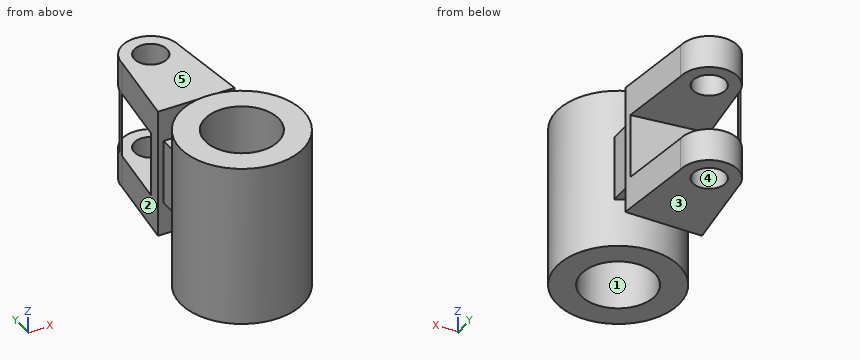
from build123d import *

# Parameters (mm, degrees)
SKETCH1_R           = 37.5
SKETCH1_R_2         = 22.5
BOSS_EXTRUDE1_DEPTH = 50
BOSS_EXTRUDE3_DEPTH = 40
SKETCH10_R          = 10
CUT_EXTRUDE5_DEPTH  = 91
SKETCH11_W          = 40
SKETCH11_H          = 59.943754609
CUT_EXTRUDE6_DEPTH  = 71.990693952
SKETCH12_W          = 40
SKETCH12_H          = 20
BOSS_EXTRUDE8_DEPTH = 20


with BuildPart() as part:
    # Sketch1 → Boss-Extrude1 (new body, symmetric)
    with BuildSketch(Plane.XY):
        Circle(SKETCH1_R)
        Circle(SKETCH1_R_2, mode=Mode.SUBTRACT)
    extrude(amount=BOSS_EXTRUDE1_DEPTH, both=True)



with BuildPart() as body_2:
    # Sketch3 → Boss-Extrude3 (new body, symmetric)
    with BuildSketch(Plane.XY):
        with BuildLine():
            Line((-23.5, 50), (23.5, 50))
            Line((23.5, 50), (17.5, 100))
            ThreePointArc((17.5, 100), (0, 117.5), (-17.5, 100))
            Line((-17.5, 100), (-23.5, 50))
        make_face()
    extrude(amount=BOSS_EXTRUDE3_DEPTH, both=True)

    # Sketch10 → Cut-Extrude5 (cut, through all)
    with BuildSketch(Plane.XY.offset(40)):
        with Locations((0, 100)):
            Circle(SKETCH10_R)
    extrude(amount=-CUT_EXTRUDE5_DEPTH, mode=Mode.SUBTRACT)

    # Sketch11 → Cut-Extrude6 (cut, through all)
    with BuildSketch(Plane(origin=(-29.081230284, 3.489747634, 0), x_dir=(0, 0, 1), z_dir=(-0.992876838, 0.119145221, 0))):
        with Locations((0, 86.815806545)):
            Rectangle(SKETCH11_W, SKETCH11_H)
    extrude(amount=-CUT_EXTRUDE6_DEPTH, mode=Mode.SUBTRACT)


with BuildPart() as part_1:
    add(part.part)

    add(body_2.part)  # Boss-Extrude8 merges body 2
    # Sketch12 → Boss-Extrude8 (add, symmetric)
    with BuildSketch(Plane.XY):
        with Locations((0, 40)):
            Rectangle(SKETCH12_W, SKETCH12_H)
    extrude(amount=BOSS_EXTRUDE8_DEPTH, both=True)


solid = part_1.part
Work out the finished part from the listing and answer in its coordinate system (mm). Face numbers are marked on the shaded views. A direction names the side the tool comes from. Round coordinates to 2 decimals unless told otherwise and drop trailing zeros. Order: outer loops, then holes, each group sorted by start corner. A loop starts at its lowest first (then second) coordinate and runs counter-clockwise, first axis right, second up. Notation, with made-up numbers: M -38.5,13.25 L 10.5,13.25 A22 ccw 10.5,27.25 Z; hole C 85.5,62.25 d6. An arc over 180 degrees is marked long. Put each result on its own line as item: value. Start each with the question number.
Q1. Straight lines are drawn through the part: L1, parallel to Y at x = 0, z = 34.75; L2, parallel to Z at x = 17, y = 85; L3, parallel to Y at x = 8, z = -28. For each, find the intervals that lie inside material, in ascending order. Write a range as [from, to].
Q2. Section A-A, the plane z = 18 is taken. Write down the section's boundary in (x, y).
Q3. Section B-B, the plane y = 84.5 is taken. Write down the section's boundary in (x, z), and give its area (3 significant figures).
Q4. Section D-D, the plane x = 0 is taken. Write down the section's boundary in (y, z).
Q5. For a pull along Y with two mould halves and no side action, classify the marked faces 1, 2 and 3 as pulls with the +Y half, pulls with the -Y half, needs draft (parallel to the pull), parting line crosses it, or undercut.
Q6. Flat-ended cylindrical pins translate along their axes: pin 1 (14 mm diameter, centred on x = -4.5, y = 80.5, fed in from -Z); pin 2 (23 mm diameter, centred on x = 0, y = 100, fed in from +Z); pin 3 (3 mm diameter, centred on y = -16.5, z = 8.5, fed in from +X). Find the tip coordinate at first contact, or state that the pin passes through.
Q7. A tool of negligible diameter and unlimited length cuts with its end or side. For the marked faces 4 and 5, from which of +Z, -Z, +X, -X, +Y, -Y can it reach the whole face along a straight path? Write none if from no direction.
Q8. Section C-C, the plane z = 34 is taken. Write down the section's boundary in (x, y).
Findings below:
1. L1: y = [-37.5, -22.5], [22.5, 37.5], [50, 90], [110, 117.5]
1. L2: z = [-40, -20], [20, 40]
1. L3: y = [-36.64, -21.03], [21.03, 36.64], [50, 94], [106, 115.56]
2. outline: M -23.5,50 L -20,50 L -20,31.72 A37.5 ccw long 20,31.72 L 20,50 L 23.5,50 L 22.96,54.5 L -22.31,59.93 Z; M -17.5,100 L -17,104.14 A17.5 ccw Z; hole C 0,0 d45
3. outline: M -19.36,-40 L 19.36,-40 L 19.36,-20 L -19.36,-20 Z; M -19.36,20 L 19.36,20 L 19.36,40 L -19.36,40 Z
3. area: 1,550 mm^2
4. outline: M -37.5,-50 L -22.5,-50 L -22.5,50 L -37.5,50 Z; M 22.5,-50 L 37.5,-50 L 37.5,-20 L 50,-20 L 50,-40 L 90,-40 L 90,-20 L 57.25,-20 L 57.25,20 L 90,20 L 90,40 L 50,40 L 50,20 L 37.5,20 L 37.5,50 L 22.5,50 Z; M 110,-40 L 117.5,-40 L 117.5,-20 L 110,-20 Z; M 110,20 L 117.5,20 L 117.5,40 L 110,40 Z
5. face 1: undercut
5. face 2: pulls with the +Y half
5. face 3: needs draft
6. pin 1: stops at z = -40
6. pin 2: stops at z = 40
6. pin 3: stops at x = 34.37
7. face 4: +Z, -Z
7. face 5: +Z, +X, -X, +Y
8. outline: C 0,0 d75; M -23.5,50 L 23.5,50 L 17.5,100 A17.5 ccw -17.5,100 Z; hole C 0,0 d45; hole C 0,100 d20
